Check sheet for the modelled part. Datum: model origin and axes. Units: mm. Round coordinates to 2 decimals unless told otherwise and drop trailing zeros. Write each loop counter-clockwise with the first axis right and the second up, starting at its lowest first coordinate (ties: lowest second). Pieces come first, ordered by that corner, then holes. Notation, with made-up numbers: (-14.75, 85) -> (-2.75, 85) arc R20 cw to (-2.75, 105) -> close; hole circle Ø1 at (82.25, 88). An arc over 180 degrees is marked (long way). Write item = value, one per line.
from build123d import *

# Parameters (mm, degrees)
SKETCH1_W           = 130
SKETCH1_H           = 60
BOSS_EXTRUDE1_DEPTH = 0.8
SKETCH2_W           = 10
SKETCH2_H           = 10
SKETCH2_W_2         = 15
SKETCH2_H_2         = 15
CUT_EXTRUDE5_DEPTH  = 3
SKETCH3_R           = 1.6
SKETCH3_R_2         = 4.1
CUT_EXTRUDE6_DEPTH  = 3
SKETCH4_W           = 13
SKETCH4_H           = 6
SKETCH4_W_2         = 10
SKETCH4_W_3         = 6
CUT_EXTRUDE8_DEPTH  = 3


with BuildPart() as part:
    # Sketch1 → Boss-Extrude1 (new body)
    with BuildSketch(Plane(origin=(0, 0, 0), x_dir=(1, 0, 0), z_dir=(0, 1, 0))):
        Rectangle(SKETCH1_W, SKETCH1_H)
    extrude(amount=BOSS_EXTRUDE1_DEPTH)

    # Sketch2 → Cut-Extrude5 (cut)
    with BuildSketch(Plane(origin=(0, 0, 0), x_dir=(1, 0, 0), z_dir=(0, 1, 0))):
        with Locations((-40.048834012, -25)):
            Rectangle(SKETCH2_W, SKETCH2_H)
        with Locations((33.42564803, 25.004850698)):
            Rectangle(SKETCH2_W, SKETCH2_H)
        with Locations((-22.460867384, 22.5)):
            Rectangle(SKETCH2_W_2, SKETCH2_H_2)
    extrude(amount=CUT_EXTRUDE5_DEPTH, mode=Mode.SUBTRACT)

    # Sketch3 → Cut-Extrude6 (cut)
    with BuildSketch(Plane(origin=(0, 0.8, 0), x_dir=(1, 0, 0), z_dir=(0, 1, 0))):
        with Locations(Location((-40.185122934, -16.467769304, 0), (0, 0, 270))):
            Circle(SKETCH3_R)
        with Locations(Location((33.794766004, 14.590842962, 0), (0, 0, 270))):
            Circle(SKETCH3_R)
        with Locations(Location((-54.63600503, -24.448107178, 0), (0, 0, 270))):
            Circle(SKETCH3_R_2)
    extrude(amount=-CUT_EXTRUDE6_DEPTH, mode=Mode.SUBTRACT)

    # Sketch4 → Cut-Extrude8 (cut)
    with BuildSketch(Plane(origin=(0, 0, 0), x_dir=(1, 0, 0), z_dir=(0, 1, 0))):
        with Locations((7.547565178, 0.728562609)):
            Rectangle(SKETCH4_W, SKETCH4_H)
        with Locations((6.386143638, -11.327057027)):
            Rectangle(SKETCH4_W_2, SKETCH4_H)
        with Locations((6.830928235, -22.580107336)):
            Rectangle(SKETCH4_W_2, SKETCH4_H)
        with Locations((29.640312606, -10.519923454)):
            Rectangle(SKETCH4_W_3, SKETCH4_H)
    extrude(amount=CUT_EXTRUDE8_DEPTH, mode=Mode.SUBTRACT)


solid = part.part
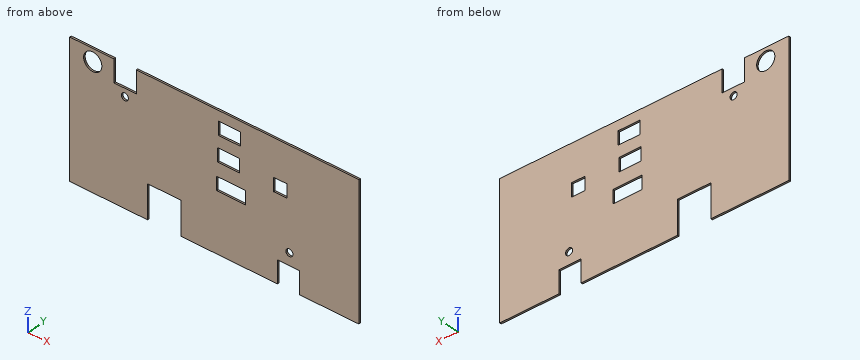
(1) Sectioned sample at B-B on x = -23.5. Enter the section's corners in (y, z), then the cut area to 3 significant figures.
Worked answers:
outline = (0, -15) -> (0.8, -15) -> (0.8, 30) -> (0, 30) -> close
area = 36.0 mm²
(2) Material ranges on L1, parallel to X at y = 0.75, z = 24; L2, parallel to X at y = 0.2, z = 13; L3, parallel to Z at x = 3, y = 0.45, recorded low to high. Write a range as [from, to].
Worked answers:
L1 = [-65, -58.71], [-50.56, -45.05], [-35.05, 1.83], [11.83, 65]
L2 = [-65, 1.39], [11.39, 26.64], [32.64, 65]
L3 = [-30, -3.73], [2.27, 8.33], [14.33, 19.58], [25.58, 30]
(3) Go/stop test with a flat-tipped pin: P1, Ø6.5, axis at x = -54.64, z = 24.45, coming from the -Y side. Record where the tip stops, or that it passes through.
Worked answers:
P1 = through
(4) Sectioned sample at A-A on y = 0.4. Count the separate pieces of the cut face and the enclosed holes in it, then the cut area to 3 significant figures.
Worked answers:
separate_pieces = 1
enclosed_holes = 7
area = 7,070 mm²
